For this review, take the finished solid that the model builds, in its own axes (mm). Give positions to 0.01 mm unless a question says otherwise; leave off trailing zeros. Order: outer loops, then holes, each group sorted by start corner. A loop starts at its lowest first (then second) coordinate and runs counter-clockwise, first axis right, second up.
from build123d import *

# Parameters (mm, degrees)
F0_R     = 31.75
F1_DEPTH = 6.35


with BuildPart() as f1:
    # F0 (on Front) → F1 (new body, symmetric)
    with BuildSketch(Plane.XZ):
        with BuildLine():
            ThreePointArc((31.851438, -12.7), (33.674842, -6.465999), (34.29, 0))
            ThreePointArc((34.29, 0), (33.674842, 6.465999), (31.851438, 12.7))
            ThreePointArc((31.851438, 12.7), (24.246692, 24.246692), (12.7, 31.851438))
            ThreePointArc((12.7, 31.851438), (6.465999, 33.674842), (0, 34.29))
            ThreePointArc((0, 34.29), (-6.465999, 33.674842), (-12.7, 31.851438))
            ThreePointArc((-12.7, 31.851438), (-24.246692, 24.246692), (-31.851438, 12.7))
            ThreePointArc((-31.851438, 12.7), (-33.674842, 6.465999), (-34.29, 0))
            ThreePointArc((-34.29, 0), (-33.674842, -6.465999), (-31.851438, -12.7))
            ThreePointArc((-31.851438, -12.7), (-24.246692, -24.246692), (-12.7, -31.851438))
            ThreePointArc((-12.7, -31.851438), (-6.465999, -33.674842), (0, -34.29))
            ThreePointArc((0, -34.29), (6.465999, -33.674842), (12.7, -31.851438))
            ThreePointArc((12.7, -31.851438), (24.246692, -24.246692), (31.851438, -12.7))
        make_face()
        Circle(F0_R, mode=Mode.SUBTRACT)
        with BuildLine():
            ThreePointArc((-34.29, 0), (-33.674842, 6.465999), (-31.851438, 12.7))
            Line((-31.851438, 12.7), (-34.29, 12.7))
            Line((-34.29, 12.7), (-34.29, 0))
        make_face()
        with BuildLine():
            Line((-34.29, -12.7), (-31.851438, -12.7))
            ThreePointArc((-31.851438, -12.7), (-33.674842, -6.465999), (-34.29, 0))
            Line((-34.29, 0), (-34.29, -12.7))
        make_face()
        with BuildLine():
            ThreePointArc((-12.7, 31.851438), (-6.465999, 33.674842), (0, 34.29))
            Line((0, 34.29), (-12.7, 34.29))
            Line((-12.7, 34.29), (-12.7, 31.851438))
        make_face()
        with BuildLine():
            ThreePointArc((0, 34.29), (6.465999, 33.674842), (12.7, 31.851438))
            Line((12.7, 31.851438), (12.7, 34.29))
            Line((12.7, 34.29), (0, 34.29))
        make_face()
        with BuildLine():
            ThreePointArc((31.851438, 12.7), (33.674842, 6.465999), (34.29, 0))
            Line((34.29, 0), (34.29, 12.7))
            Line((34.29, 12.7), (31.851438, 12.7))
        make_face()
        with BuildLine():
            Line((34.29, -12.7), (34.29, 0))
            ThreePointArc((34.29, 0), (33.674842, -6.465999), (31.851438, -12.7))
            Line((31.851438, -12.7), (34.29, -12.7))
        make_face()
        with BuildLine():
            Line((12.7, -34.29), (12.7, -31.851438))
            ThreePointArc((12.7, -31.851438), (6.465999, -33.674842), (0, -34.29))
            Line((0, -34.29), (12.7, -34.29))
        make_face()
        with BuildLine():
            Line((-12.7, -34.29), (0, -34.29))
            ThreePointArc((0, -34.29), (-6.465999, -33.674842), (-12.7, -31.851438))
            Line((-12.7, -31.851438), (-12.7, -34.29))
        make_face()
    extrude(amount=F1_DEPTH, both=True)


solid = f1.part
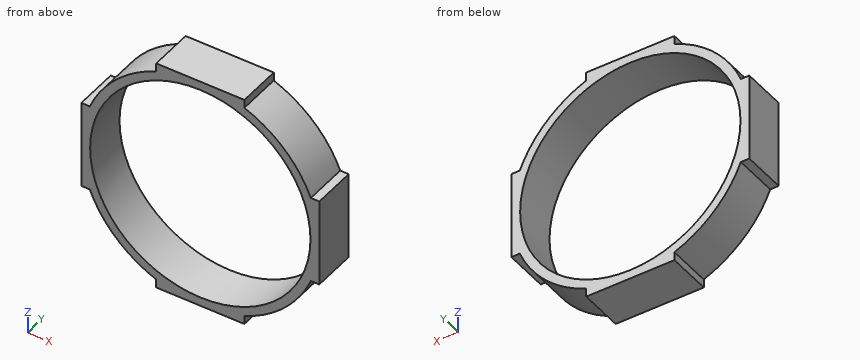
1) Clearance check with flat-ended pins moving along their axes: pin 1 (1.2 mm diameter, centred on y = -3, z = -33.5, fed in from +X); pin 2 (0.7 mm diameter, centred on x = 33, y = -1, fed in from -Z); pin 3 (1.5 mm diameter, centred on x = -18, y = -2.5, fed in from +Z). State where each tip first meets the part, or that it passes through.
Answer sheet:
pin 1: stops at x = 12.7
pin 2: stops at z = -12.7
pin 3: stops at z = 29.64
2) We need section C-C on z = 14.5. Give the boundary of the cut face in (x, y), then the cut area to 3 significant figures.
Answer sheet:
outline: (-31.07, -6.35) - (-28.25, -6.35) - (-28.25, 6.35) - (-31.07, 6.35) - close; (28.25, -6.35) - (31.07, -6.35) - (31.07, 6.35) - (28.25, 6.35) - close
area: 71.8 mm2
3) To check wall thickness, follow line 1 (Z direction, x = 1, y = 1.75); line 2 (Z direction, x = -2.5, y = -3.25); line 3 (X direction, y = -4.5, z = -16). State the ranges of each line that lie inside material, in increasing order.
Answer sheet:
line 1: z = -34.29 to -31.73, 31.73 to 34.29
line 2: z = -34.29 to -31.65, 31.65 to 34.29
line 3: x = -30.33 to -27.42, 27.42 to 30.33
4) We need section A-A on x = 0. Give the boundary of the cut face in (y, z).
Answer sheet:
outline: (-6.35, -34.29) - (6.35, -34.29) - (6.35, -31.75) - (-6.35, -31.75) - close; (-6.35, 31.75) - (6.35, 31.75) - (6.35, 34.29) - (-6.35, 34.29) - close
5) We need section B-B on y = -3. Give the boundary of the cut face in (x, z).
Answer sheet:
outline: (-34.29, -12.7) - (-31.85, -12.7) arc R34.29 ccw to (-12.7, -31.85) - (-12.7, -34.29) - (12.7, -34.29) - (12.7, -31.85) arc R34.29 ccw to (31.85, -12.7) - (34.29, -12.7) - (34.29, 12.7) - (31.85, 12.7) arc R34.29 ccw to (12.7, 31.85) - (12.7, 34.29) - (-12.7, 34.29) - (-12.7, 31.85) arc R34.29 ccw to (-31.85, 12.7) - (-34.29, 12.7) - close; hole circle Ø63.5 at (0, 0)
